Source: three-view drawing plus pictorial views. Frame: mm from the lowest corner of the part. A direction names the side the tool comes from. Coordinates: 2 decimals unless noted, no trailing zeros. Order: outer loops, then holes, each group sorted by start corner. A loop starts at its lowest first (then second) coordinate and runs counter-clockwise, first axis right, second up. Notation, with made-up numbers: M 13.5,86 L 46.5,86 A22 cw 46.5,106 Z; hole C 88.25,-39 d10. An arc over 180 degrees is marked long. One line per question, with ' | ' between items.
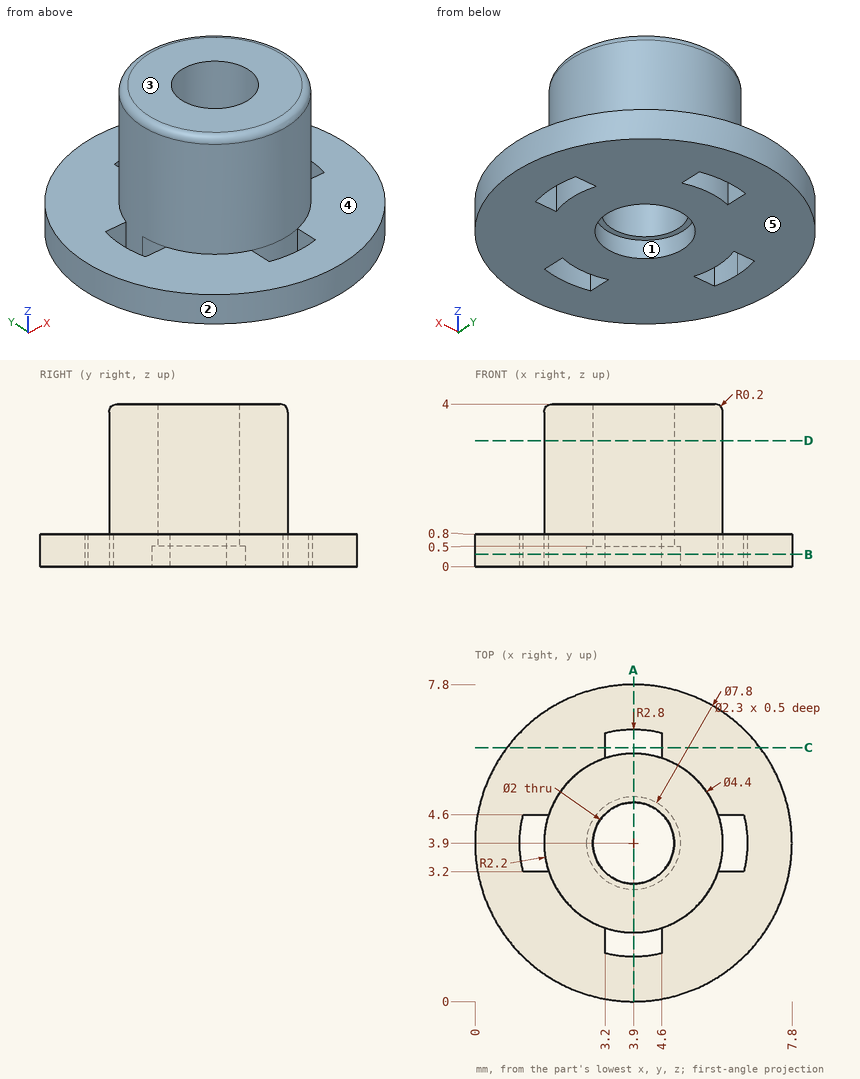
1. Material intervals for line 1 (Y direction, x = 3.9, z = 0.35); line 2 (Y direction, x = 3.9, z = 3.1), sorted ascending. Write a range as [from, to].
Response values:
line 1: y = [0, 1.1], [1.7, 2.75], [5.05, 6.1], [6.7, 7.8] | line 2: y = [1.7, 2.9], [4.9, 6.1]
2. Section C-C, the plane y = 6.25. Output: boundary loops of the cut face in (x, z), and give its area (3 significant figures).
Response values:
outline: M 0.79,0 L 3.2,0 L 3.2,0.8 L 0.79,0.8 Z; M 4.6,0 L 7.01,0 L 7.01,0.8 L 4.6,0.8 Z | area: 3.86 mm^2
3. Section D-D, the plane z = 3.1. Output: boundary loops of the cut face in (x, y).
Response values:
outline: C 3.9,3.9 d4.4; hole C 3.9,3.9 d2
4. Section A-A, the plane x = 3.9. Output: boundary loops of the cut face in (y, z), and give its area (3 significant figures).
Response values:
outline: M 0,0 L 1.1,0 L 1.1,0.8 L 0,0.8 Z; M 1.7,0 L 2.75,0 L 2.75,0.5 L 2.9,0.5 L 2.9,4 L 1.9,4 A0.2 ccw 1.7,3.8 Z; M 4.9,0.5 L 5.05,0.5 L 5.05,0 L 6.1,0 L 6.1,3.8 A0.2 ccw 5.9,4 L 4.9,4 Z; M 6.7,0 L 7.8,0 L 7.8,0.8 L 6.7,0.8 Z | area: 11.2 mm^2
5. Access query for the marked faces 4 and 5. Directions: +Z, -Z, +X, -X, +Y, -Y. A direction counts if a zero-diameter tool reaches every point of the face in a straight line with its end or side. Return the directions, or none.
Response values:
face 4: +Z | face 5: -Z, +X, -X, +Y, -Y
6. Draft query along X for the marked faces 1, 2 and 3. Return one class per face: pulls with the +X half, pulls with the -X half, needs draft (parallel to the pull), parting line crosses it, or undercut.
Response values:
face 1: undercut | face 2: parting line crosses it | face 3: needs draft
7. Section B-B, the plane z = 0.3. Output: boundary loops of the cut face in (x, y).
Response values:
outline: C 3.9,3.9 d7.8; hole M 1.19,3.2 L 1.81,3.2 A2.2 cw 1.81,4.6 L 1.19,4.6 A2.8 ccw Z; hole C 3.9,3.9 d2.3; hole M 3.2,1.19 A2.8 ccw 4.6,1.19 L 4.6,1.81 A2.2 cw 3.2,1.81 Z; hole M 3.2,5.99 A2.2 cw 4.6,5.99 L 4.6,6.61 A2.8 ccw 3.2,6.61 Z; hole M 5.99,3.2 L 6.61,3.2 A2.8 ccw 6.61,4.6 L 5.99,4.6 A2.2 cw Z
8. Pin query (flat end, axial travel): P1, Ø0.5, axis at x = 6.5, z = 0, coming from the +Y side; P2, Ø2.5, axis at x = 3.5, y = 3.5, coming from the +Z side; P3, Ø1.6, axis at x = 3.9, y = 3.9, coming from the +Z side. Return the tip coordinate at first contact, or that it passes through.
Response values:
P1: stops at y = 7.01 | P2: stops at z = 4 | P3: passes through
